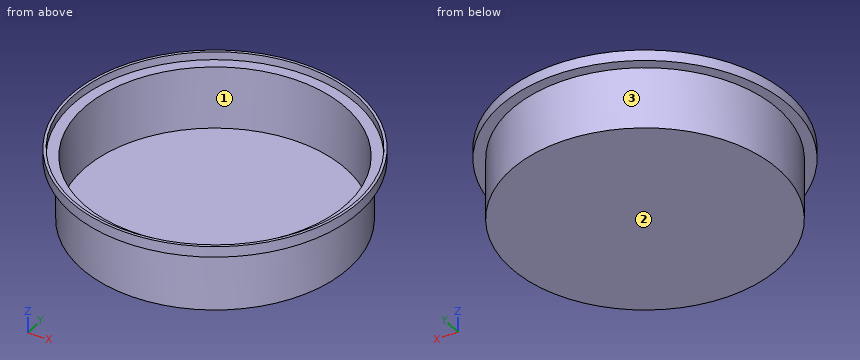
from build123d import *

# Parameters (mm, degrees)
F2_T     = -1.27
F3_R     = 62.23
F4_DEPTH = 0.47


with BuildPart() as f1:
    # F0 (on Front) → F1 (revolve)
    with BuildSketch(Plane.XZ):
        Polygon((0, 34.29), (0, 0), (63.5, 0), (63.5, 29.21), (68.58, 29.21), (68.58, 34.29), align=None)
    revolve(axis=Axis((0, 0, -14.2717824864), (0, 0, -1)))

    # F2
    f2_openings = [f1.faces().sort_by_distance(p)[0] for p in [
        (0, 0, 34.29),
    ]]
    offset(amount=F2_T, openings=f2_openings, kind=Kind.INTERSECTION)

    # F3 (on face) → F4 (cut, through all)
    with BuildSketch(Plane.XY.offset(1.27)):
        Circle(F3_R)
    extrude(amount=-F4_DEPTH, mode=Mode.SUBTRACT)


solid = f1.part
Verification items for the finished model (mm, model axes). Face numbers are marked on the shaded views. Coordinates: 2 decimals unless noted, no trailing zeros. Loops run counter-clockwise (first coordinate to the right, second up) from the corner with the lowest first, then second, coordinate; pieces in that order, holes last. Notation, with made-up numbers: M 85.5,-35.5 L 135.5,-35.5 A14 ccw 135.5,-22.5 Z; hole C -8,39.25 d1. An arc over 180 degrees is marked long. One line per item, written item: value.
1. Gauge pin test, flat ends, axial feed: P1, Ø1.5, axis at x = 49, y = 36, coming from the +Z side; P2, Ø1.5, axis at x = -51.5, z = 30.5, coming from the +Y side; P3, Ø12, axis at x = -16, z = 17, coming from the +Y side. Record the tip position at first contact, or that the pin passes through.
Answers follow:
P1: z = 0.8
P2: y = 46.13
P3: y = 62.71
2. Section check A-A on z = 23.5. Record the cut outline in (x, y).
Answers follow:
outline: C 0,0 d127; hole C 0,0 d124.46
3. Material ranges on line 1 along Y through (x, z) = (0, 9); line 2 along Y through (x, z) = (0, 31.75); line 3 along Z through (x, y) = (-53.5, -37), recorded low to high. Write a range as from..to.
Answers follow:
line 1: -63.5..-62.23, 62.23..63.5
line 2: -68.58..-67.31, 67.31..68.58
line 3: 29.21..30.48
4. Mould release check, pull along Y, two halves, no side actions. Record for the marked faces 1, 2 and 3: pulls with the +Y half, pulls with the -Y half, needs draft (parallel to the pull), parting line crosses it, or undercut.
Answers follow:
face 1: undercut
face 2: needs draft
face 3: parting line crosses it
5. Section check B-B on y = 31. Record the cut outline in (x, z).
Answers follow:
outline: M -61.17,29.21 L -55.42,29.21 L -55.42,0 L 55.42,0 L 55.42,29.21 L 61.17,29.21 L 61.17,34.29 L 59.75,34.29 L 59.75,30.48 L 53.96,30.48 L 53.96,0.8 L -53.96,0.8 L -53.96,30.48 L -59.75,30.48 L -59.75,34.29 L -61.17,34.29 Z
6. Section check C-C on x = 0. Record the cut outline in (y, z).
Answers follow:
outline: M -68.58,29.21 L -63.5,29.21 L -63.5,0 L 63.5,0 L 63.5,29.21 L 68.58,29.21 L 68.58,34.29 L 67.31,34.29 L 67.31,30.48 L 62.23,30.48 L 62.23,0.8 L -62.23,0.8 L -62.23,30.48 L -67.31,30.48 L -67.31,34.29 L -68.58,34.29 Z
